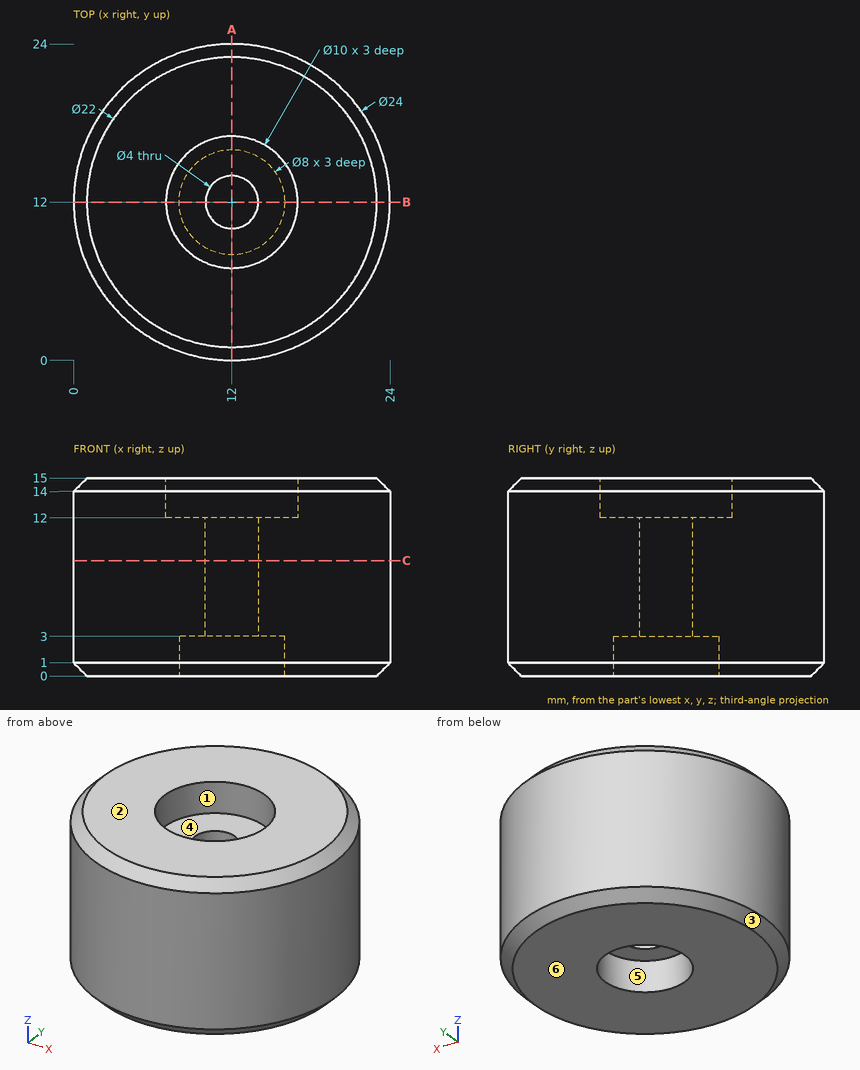
Check sheet for the drawn part. Datum: minimum x, y, z corner. Units: mm. A direction names the side the tool comes from. Give positions to 0.01 mm unless a question says otherwise; leave off trailing zeros. Order: outer loops, then holes, each group sorted by start corner. A loop starts at its lowest first (then second) coordinate and runs counter-clockwise, first axis right, second up. Notation, with made-up numbers: (28, -24.5) -> (80, -24.5) arc R25 ccw to (80, 5.5) -> close; hole circle Ø5 at (26.25, 21). An arc over 180 degrees is marked (long way). Return JSON: item names as keys, results as strings.
1. Material ranges on probe 1 along Y at (x, z) = (12, 1.4); probe 2 along Y at (x, z) = (12, 12.85); probe 3 along Z at (x, y) = (11.5, 14.25), recorded low to high. Write a range as [from, to].
From the geometry:
{"probe 1": "[0, 8], [16, 24]", "probe 2": "[0, 7], [17, 24]", "probe 3": "[3, 12]"}
2. Cross-section at A-A, the plane x = 12. Record the cut outline in (y, z).
From the geometry:
{"outline": "(0, 1) -> (1, 0) -> (8, 0) -> (8, 3) -> (10, 3) -> (10, 12) -> (7, 12) -> (7, 15) -> (1, 15) -> (0, 14) -> close; (14, 3) -> (16, 3) -> (16, 0) -> (23, 0) -> (24, 1) -> (24, 14) -> (23, 15) -> (17, 15) -> (17, 12) -> (14, 12) -> close"}
3. Cross-section at C-C, the plane z = 8.75. Record the cut outline in (x, y).
From the geometry:
{"outline": "circle Ø24 at (12, 12); hole circle Ø4 at (12, 12)"}
4. Set-up check for the marked faces 5 and 6: record each of +Z, -Z, +X, -X, +Y, -Y from which the full face is reachable in a straight line by a thin tool's end or side.
From the geometry:
{"face 5": "-Z", "face 6": "-Z, +X, -X, +Y, -Y"}
5. Mould release check, pull along X, two halves, no side actions. Record for the marked faces 1, 2, 3 and 4: +X half, -X half, draft (parallel to the pull), parting line (faces both ways), or undercut.
From the geometry:
{"face 1": "undercut", "face 2": "draft", "face 3": "parting line", "face 4": "undercut"}
6. Go/stop test with flat-tipped pins: P1, Ø3, axis at x = 12, y = 12, coming from the -Z side (3 decimals); P2, Ø5, axis at y = 9, z = 7.5, coming from the -X side; P3, Ø5, axis at x = 12, y = 12, coming from the +Z side; P4, Ø6.5, axis at x = 13.5, y = 10, coming from the -Z side. Record where each tip stops, or that it passes through.
From the geometry:
{"P1": "through", "P2": "x = 0.01", "P3": "z = 12", "P4": "z = 0"}
